Autodesk Inventor part; units mm, degrees
ref_plane "YZ Plane" through (0, 0, 0) normal (1, 0, 0) x (0, 1, 0)
ref_plane "XZ Plane" through (0, 0, 0) normal (0, 1, 0) x (-1, 0, 0)
ref_plane "XY Plane" through (0, 0, 0) normal (0, 0, 1) x (1, 0, 0)
sketch "Sketch1" plane through (0, 0, 0) normal (1, 0, 0) x (0, 1, 0)
  line L0 (-20, -20) -> (20, -20)
  line L1 (20, -20) -> (20, 20)
  line L2 (20, 20) -> (-20, 20)
  line L3 (-20, 20) -> (-20, -20)
  line L4 (-20, -20) -> (20, 20) construction
  line L5 (20, -20) -> (-20, 20) construction
  point P0 (0, 0)
  dimension "d1" = 40
  dimension "d2" = 40
extrude "Outline" add sketch "Sketch1" along normal blind 2.5
sketch "Sketch2" plane through (2.5, 0, 0) normal (1, 0, 0) x (0, 0, -1)
  line L0 (20, 20) -> (-20, 20)
  line L1 (20, -20) -> (20, 20)
  line L2 (-18, 3.1) -> (-13, 3.1)
  line L3 (-13, 3.1) -> (-13, -3.1)
  line L4 (-13, -3.1) -> (-18, -3.1)
  line L5 (-18, -3.1) -> (-18, 3.1)
  line L6 (-11, 0.75) -> (-4.4788, 0.75)
  line L7 (-4.4788, 0.75) -> (-4.4788, -0.75)
  line L8 (-4.4788, -0.75) -> (-11, -0.75)
  line L9 (-11, -0.75) -> (-11, 0.75)
  line L10 (13.9738, 2.8192) -> (18, 0)
  line L11 (18, 0) -> (13.9738, -2.8192)
  line L12 (13.9738, 2.8192) -> (13.4003, 2)
  line L13 (13.4003, 2) -> (16.2566, 0)
  line L14 (16.2566, 0) -> (13.4003, -2)
  line L15 (13.4003, -2) -> (13.9738, -2.8192)
  line L16 (-18, 0) -> (16.2566, 0) construction
  arc A0 (14.0039, 1.5773) -> (14.0039, -1.5773) centre (16.2566, 0) ccw
  arc A1 (14.823, 1.0038) -> (14.823, -1.0038) centre (16.2566, 0) ccw
  line L17 (4.9853, 0.75) -> (11.5066, 0.75)
  line L18 (11.5066, 0.75) -> (11.5066, -0.75)
  line L19 (11.5066, -0.75) -> (4.9853, -0.75)
  line L20 (4.9853, -0.75) -> (4.9853, 0.75)
  line L21 (-11.3236, 2.0044) -> (-11.048, 1.0432)
  line L22 (-11.048, 1.0432) -> (-7.203, 2.1457)
  line L23 (-7.203, 2.1457) -> (-7.4786, 3.107)
  line L24 (-7.4786, 3.107) -> (-11.3236, 2.0044)
  line L25 (-11.048, -1.0432) -> (-7.203, -2.1457)
  line L26 (-7.203, -2.1457) -> (-7.4786, -3.107)
  line L27 (-7.4786, -3.107) -> (-11.3236, -2.0044)
  line L28 (-11.3236, -2.0044) -> (-11.048, -1.0432)
  circle A2 centre (-16.5, 0) radius 5.5509 construction
  line L29 (-11.9623, 3.1972) -> (-11.4623, 2.3312)
  line L30 (-11.4623, 2.3312) -> (-9.2973, 3.5812)
  line L31 (-9.2973, 3.5812) -> (-9.7973, 4.4472)
  line L32 (-9.7973, 4.4472) -> (-11.9623, 3.1972)
  line L33 (-11.4623, -2.3312) -> (-11.9623, -3.1972)
  line L34 (-11.9623, -3.1972) -> (-9.7973, -4.4472)
  line L35 (-9.7973, -4.4472) -> (-9.2973, -3.5812)
  line L36 (-9.2973, -3.5812) -> (-11.4623, -2.3312)
  line L37 (-4.9984, 6.0961) -> (-2.4003, 7.5961)
  line L38 (-2.4003, 7.5961) -> (5.5049, -6.0961)
  line L39 (5.5049, -6.0961) -> (2.9068, -7.5961)
  line L40 (2.9068, -7.5961) -> (-4.9984, 6.0961)
  line L41 (-4.9984, -6.0961) -> (2.9068, 7.5961)
  line L42 (2.9068, 7.5961) -> (5.5049, 6.0961)
  line L43 (5.5049, 6.0961) -> (-2.4003, -7.5961)
  line L44 (-2.4003, -7.5961) -> (-4.9984, -6.0961)
  line L45 (-4.9984, 7.5961) -> (5.5049, 7.5961) construction
  line L46 (5.5049, 7.5961) -> (5.5049, -7.5961) construction
  line L47 (5.5049, -7.5961) -> (-4.9984, -7.5961) construction
  line L48 (-4.9984, -7.5961) -> (-4.9984, 7.5961) construction
  line L49 (-20, -20) -> (20, -20)
  line L50 (-20, 20) -> (-20, -20)
  line L51 (-4.9984, 6.0961) -> (-11, 6.0961) construction
  line L52 (5.5049, 6.0961) -> (11.5066, 6.0961) construction
  point P0 (0, 0)
  point P1 (-13, 0)
  point P2 (-11, 0)
  point P3 (13.5066, 0)
  point P4 (-1.0458, 0.75)
  point P5 (1.5523, 0.75)
  point P6 (0.2533, -7.5961)
  point P7 (11.5066, 0)
  point P8 (5.5049, 0)
  point P9 (4.9853, 0)
  point P10 (-1.4788, 0)
  point P11 (0.2533, -3)
  point P12 (1.9853, 0)
  point P13 (0.2533, 3)
  point P14 (20, 0)
  dimension "d12" = 35
  dimension "d13" = 35
  dimension "d14" = 4
  dimension "d15" = 1
  dimension "d16" = 1
  dimension "d17" = 2.75
  dimension "d18" = 1.5
  dimension "d19" = 2
  dimension "d21" = 5
  dimension "d22" = 2
  dimension "d23" = 1
  dimension "d24" = 1
  dimension "d25" = 3.5
  dimension "d26" = 16
  dimension "d27" = 16
  dimension "d28" = 4
  dimension "d29" = 2.5
  dimension "d30" = 1
  dimension "d31" = 14
  dimension "d32" = 14
  dimension "d33" = 1
  dimension "d34" = 2.5
  dimension "d35" = 6.2
  dimension "d36" = 60
  dimension "d37" = 60
  dimension "d38" = 3
  dimension "d40" = 2
  dimension "d41" = 2
  dimension "d42" = 3
  dimension "d45" = 15.1922
extrude "Extrusion2" cut sketch "Sketch2" against normal blind 1 contours L2 L3 L4 L5 | L6 L7 L8 L9 | L10 L11 L15 L14 L13 L12 | L13 A1 L14 A0 | L17 L18 L19 L20 | L24 L23 L22 L21 | L25 L26 L27 L28 | L32 L31 L30 L29 | L36 L35 L34 L33 | L37 L38 L41 L40 | L41 L38 L43 L40 | L40 L43 L44 L41 | L41 L42 L43 L38 | L43 L38 L39 L40
sketch "Sketch4" plane through (1.5, 0, 0) normal (1, 0, 0) x (0, 0, -1)
  line L0 (-11.3236, 2.0044) -> (-11.048, 1.0432)
  line L1 (-11.048, 1.0432) -> (-7.203, 2.1457)
  line L2 (-7.203, 2.1457) -> (-7.4786, 3.107)
  line L3 (-7.4786, 3.107) -> (-11.3236, 2.0044)
  line L4 (0.2533, -3) -> (2.9068, -7.5961)
  line L5 (2.9068, -7.5961) -> (5.5049, -6.0961)
  line L6 (5.5049, -6.0961) -> (1.9853, 0)
  line L7 (1.9853, 0) -> (5.5049, 6.0961)
  line L8 (5.5049, 6.0961) -> (2.9068, 7.5961)
  line L9 (2.9068, 7.5961) -> (0.2533, 3)
  line L10 (0.2533, 3) -> (-2.4003, 7.5961)
  line L11 (-2.4003, 7.5961) -> (-4.9984, 6.0961)
  line L12 (-4.9984, 6.0961) -> (-1.4788, 0)
  line L13 (-1.4788, 0) -> (-4.9984, -6.0961)
  line L14 (-4.9984, -6.0961) -> (-2.4003, -7.5961)
  line L15 (-2.4003, -7.5961) -> (0.2533, -3)
  line L16 (11.5066, 0.75) -> (4.9853, 0.75)
  line L17 (4.9853, 0.75) -> (4.9853, -0.75)
  line L18 (4.9853, -0.75) -> (11.5066, -0.75)
  line L19 (11.5066, -0.75) -> (11.5066, 0.75)
  line L20 (-9.2973, 3.5812) -> (-9.7973, 4.4472)
  line L21 (-9.7973, 4.4472) -> (-11.9623, 3.1972)
  line L22 (-11.9623, 3.1972) -> (-11.4623, 2.3312)
  line L23 (-11.4623, 2.3312) -> (-9.2973, 3.5812)
  line L24 (-4.4788, -0.75) -> (-4.4788, 0.75)
  line L25 (-4.4788, 0.75) -> (-11, 0.75)
  line L26 (-11, 0.75) -> (-11, -0.75)
  line L27 (-11, -0.75) -> (-4.4788, -0.75)
  line L28 (-9.7973, -4.4472) -> (-9.2973, -3.5812)
  line L29 (-9.2973, -3.5812) -> (-11.4623, -2.3312)
  line L30 (-11.4623, -2.3312) -> (-11.9623, -3.1972)
  line L31 (-11.9623, -3.1972) -> (-9.7973, -4.4472)
  line L32 (14.823, 1.0038) -> (16.2566, 0)
  line L33 (16.2566, 0) -> (14.823, -1.0038)
  arc A0 (14.823, 1.0038) -> (14.823, -1.0038) centre (16.2566, 0) ccw
  line L34 (13.9738, -2.8192) -> (18, 0)
  line L35 (18, 0) -> (13.9738, 2.8192)
  line L36 (13.9738, 2.8192) -> (13.4003, 2)
  line L37 (13.4003, 2) -> (14.0039, 1.5773)
  arc A1 (14.0039, 1.5773) -> (14.0039, -1.5773) centre (16.2566, 0) ccw
  line L38 (14.0039, -1.5773) -> (13.4003, -2)
  line L39 (13.4003, -2) -> (13.9738, -2.8192)
  line L40 (-11.3236, -2.0044) -> (-7.4786, -3.107)
  line L41 (-7.4786, -3.107) -> (-7.203, -2.1457)
  line L42 (-7.203, -2.1457) -> (-11.048, -1.0432)
  line L43 (-11.048, -1.0432) -> (-11.3236, -2.0044)
  line L44 (-13, -3.1) -> (-13, 3.1)
  line L45 (-13, 3.1) -> (-18, 3.1)
  line L46 (-18, 3.1) -> (-18, -3.1)
  line L47 (-18, -3.1) -> (-13, -3.1)
  line L48 (20, 20) -> (20, -20)
  line L49 (20, -20) -> (-20, -20)
  line L50 (-20, -20) -> (-20, 20)
  line L51 (-20, 20) -> (20, 20)
  point P0 (0, 0)
fillet "Fillet1" radius 5 4 edges at (1.25, 20, -20) (1.25, -20, -20) (1.25, 20, 20) (1.25, -20, 20)
sketch "Sketch5" plane through (2.5, 0, 0) normal (1, 0, 0) x (0, 0, -1)
  arc A0 (-20, -15) -> (-15, -20) centre (-15, -15) ccw
  line L0 (-20, -15) -> (-20, 15)
  arc A1 (-15, 20) -> (-20, 15) centre (-15, 15) ccw
  line L1 (-15, 20) -> (15, 20)
  arc A2 (20, 15) -> (15, 20) centre (15, 15) ccw
  line L2 (20, 15) -> (20, -15)
  arc A3 (15, -20) -> (20, -15) centre (15, -15) ccw
  line L3 (15, -20) -> (-15, -20)
  line L4 (-13, -3.1) -> (-13, 3.1)
  line L5 (-13, 3.1) -> (-18, 3.1)
  line L6 (-18, 3.1) -> (-18, -3.1)
  line L7 (-18, -3.1) -> (-13, -3.1)
  line L8 (-11.3236, -2.0044) -> (-7.4786, -3.107)
  line L9 (-7.4786, -3.107) -> (-7.203, -2.1457)
  line L10 (-7.203, -2.1457) -> (-11.048, -1.0432)
  line L11 (-11.048, -1.0432) -> (-11.3236, -2.0044)
  line L12 (13.9738, -2.8192) -> (18, 0)
  line L13 (18, 0) -> (13.9738, 2.8192)
  line L14 (13.9738, 2.8192) -> (13.4003, 2)
  line L15 (13.4003, 2) -> (14.0039, 1.5773)
  arc A4 (14.0039, 1.5773) -> (14.0039, -1.5773) centre (16.2566, 0) ccw
  line L16 (14.0039, -1.5773) -> (13.4003, -2)
  line L17 (13.4003, -2) -> (13.9738, -2.8192)
  line L18 (-9.7973, -4.4472) -> (-9.2973, -3.5812)
  line L19 (-9.2973, -3.5812) -> (-11.4623, -2.3312)
  line L20 (-11.4623, -2.3312) -> (-11.9623, -3.1972)
  line L21 (-11.9623, -3.1972) -> (-9.7973, -4.4472)
  line L22 (-4.4788, -0.75) -> (-4.4788, 0.75)
  line L23 (-4.4788, 0.75) -> (-11, 0.75)
  line L24 (-11, 0.75) -> (-11, -0.75)
  line L25 (-11, -0.75) -> (-4.4788, -0.75)
  line L26 (-9.2973, 3.5812) -> (-9.7973, 4.4472)
  line L27 (-9.7973, 4.4472) -> (-11.9623, 3.1972)
  line L28 (-11.9623, 3.1972) -> (-11.4623, 2.3312)
  line L29 (-11.4623, 2.3312) -> (-9.2973, 3.5812)
  line L30 (11.5066, 0.75) -> (4.9853, 0.75)
  line L31 (4.9853, 0.75) -> (4.9853, -0.75)
  line L32 (4.9853, -0.75) -> (11.5066, -0.75)
  line L33 (11.5066, -0.75) -> (11.5066, 0.75)
  line L34 (0.2533, -3) -> (2.9068, -7.5961)
  line L35 (2.9068, -7.5961) -> (5.5049, -6.0961)
  line L36 (5.5049, -6.0961) -> (1.9853, 0)
  line L37 (1.9853, 0) -> (5.5049, 6.0961)
  line L38 (5.5049, 6.0961) -> (2.9068, 7.5961)
  line L39 (2.9068, 7.5961) -> (0.2533, 3)
  line L40 (0.2533, 3) -> (-2.4003, 7.5961)
  line L41 (-2.4003, 7.5961) -> (-4.9984, 6.0961)
  line L42 (-4.9984, 6.0961) -> (-1.4788, 0)
  line L43 (-1.4788, 0) -> (-4.9984, -6.0961)
  line L44 (-4.9984, -6.0961) -> (-2.4003, -7.5961)
  line L45 (-2.4003, -7.5961) -> (0.2533, -3)
  line L46 (-11.3236, 2.0044) -> (-11.048, 1.0432)
  line L47 (-11.048, 1.0432) -> (-7.203, 2.1457)
  line L48 (-7.203, 2.1457) -> (-7.4786, 3.107)
  line L49 (-7.4786, 3.107) -> (-11.3236, 2.0044)
  line L50 (14.823, 1.0038) -> (16.2566, 0)
  line L51 (16.2566, 0) -> (14.823, -1.0038)
  arc A5 (14.823, 1.0038) -> (14.823, -1.0038) centre (16.2566, 0) ccw
  point P0 (0, 0)
properties part number "LightGateCard_3DPrint"
Input: part model. Units: mm. Frame: model coordinates. A direction names the side the tool comes from. Coordinates: 2 decimals unless noted, no trailing zeros. Write each loop counter-clockwise with the first axis right and the second up, starting at its lowest first coordinate (ties: lowest second). Pieces come first, ordered by that corner, then holes. Notation, with made-up numbers: (74.25, 58.5) - (86.25, 58.5) arc R19 cw to (86.25, 65.5) - close; hole circle Ø6 at (81.25, -29.75). An arc over 180 degrees is marked (long way). Put each result on its own line as item: value. Start each with the question number.
1) Contact query for flat-ended pins moving along their axis: pin 1 (0.5 mm diameter, centred on x = 2, z = 16.5, fed in from +Y); pin 2 (0.5 mm diameter, centred on x = 2, z = 15.5, fed in from -Y). Output: stop coordinate, or through.
2) Cut plane B-B (x = 1.9). State how many separate pieces and enclosed holes the cut face has, plus the area to 3 significant figures.
3) Ray query, L1, parallel to Y at x = 2.45, z = 7.5; L2, parallel to Y at x = 2.2, z = 13.5; L3, parallel to Y at x = 2.25, z = 9. Return the intervals inside material, ascending.
4) Cut plane A-A (z = -7). Return the cut outline in (x, y).
5) Reachability of faces 4 (the face through (2, 3.1, 16)), 5 (the face through (1, -18, 19)) from +Z, -Z, +X, -X, +Y, -Y: full face, straight path, thin tool, end or side. Return the list, or none.
6) Mould query, pull axis Y, two halves, no side actions, for faces 1 (the face through (1.5, 0, 0)), 2 (the face through (2.007, 6.836, 3.718)), 3 (the face through (1, -20, 0)). Classes: pulls with the +Y half, pulls with the -Y half, needs draft (parallel to the pull), parting line crosses it, or undercut.
Resolved:
1. pin 1: stops at y = 19.84
1. pin 2: stops at y = -19.99
2. separate pieces: 2
2. enclosed holes: 9
2. area: 1,420 mm2
3. L1: y = -20 to -3.1, -2.06 to -0.75, 0.75 to 2.06, 3.1 to 20
3. L2: y = -20 to -3.1, 3.1 to 20
3. L3: y = -20 to -2.67, -1.63 to -0.75, 0.75 to 1.63, 2.67 to 20
4. outline: (0, -20) - (2.5, -20) - (2.5, -0.75) - (1.5, -0.75) - (1.5, 0.75) - (2.5, 0.75) - (2.5, 20) - (0, 20) - close
5. face 4: +X
5. face 5: +Z, +X, -X, -Y
6. face 1: undercut
6. face 2: undercut
6. face 3: pulls with the -Y half
